Could you check a few things on this model? Use its own coordinates, in mm. A direction names the side the tool comes from. Round coordinates to 2 decimals unless told otherwise and drop trailing zeros. Loops run counter-clockwise (first coordinate to the right, second up) from the corner with the lowest first, then second, coordinate; pieces in that order, holes last. Notation, with made-up numbers: (29, -30.75) - (84, -30.75) arc R13 cw to (84, -26.75) - close; hole circle Ø2 at (83.5, -10.5). An arc over 180 degrees is marked (long way). Use one line per item in the form item = value.
```python
from build123d import *

# Parameters (mm, degrees)
F0_R     = 8.001
F0_R_2   = 1.27
F1_DEPTH = 31.75
F2_R     = 2.413
F2_R_2   = 1.27
F3_DEPTH = 19.05
F4_R     = 2.159
F5_DEPTH = 12.7
F6_DEPTH = 12.7


with BuildPart() as f1:
    # F0 (on Top) → F1 (new body)
    with BuildSketch(Plane.XY):
        Circle(F0_R)
        Circle(F0_R_2, mode=Mode.SUBTRACT)
    extrude(amount=F1_DEPTH)

    # F2 (on face) → F3 (cut)
    with BuildSketch(Plane.XY.offset(31.75)):
        Circle(F2_R)
        Circle(F2_R_2, mode=Mode.SUBTRACT)
    extrude(amount=-F3_DEPTH, mode=Mode.SUBTRACT)

    # F4 (on Right) → F5 (cut, symmetric)
    with BuildSketch(Plane.YZ):
        with Locations((0, 20.955)):
            Circle(F4_R)
    extrude(amount=F5_DEPTH, both=True, mode=Mode.SUBTRACT)

    # F4 (on Right) → F6 (cut, symmetric)
    with BuildSketch(Plane.YZ):
        with Locations((0, 6.35)):
            Circle(F4_R)
    extrude(amount=F6_DEPTH, both=True, mode=Mode.SUBTRACT)


solid = f1.part
```
1. Please list where these lines run through material, in increasing order: line 1 along Z through (x, y) = (6.75, 0); line 2 along Y through (x, z) = (0, 2.65).
Solution:
line_1 = 0 to 4.19, 8.51 to 18.8, 23.11 to 31.75
line_2 = -8 to -1.27, 1.27 to 8
2. We'd pull the mould along Y, two halves only. Please class faces 1 (the face through (1.04, -1.04, 12.7)), 2 (the face through (2, 0, 0)), 3 (the face through (-1.27, 0.06, 2.27)), 4 (the face through (7.632, 2.403, 15.653)): +Y half, -Y half, draft (parallel to the pull), parting line (faces both ways), or undercut.
Solution:
face_1 = undercut
face_2 = draft
face_3 = undercut
face_4 = parting line
3. If we section it at A-A, the plane y = 0: Write out the boundary of the cut face in (x, z), plus the area to 3 significant figures.
Solution:
outline = (-8, 0) - (-1.27, 0) - (-1.27, 4.19) - (-8, 4.19) - close; (-8, 8.51) - (-1.27, 8.51) - (-1.27, 12.7) - (-2.41, 12.7) - (-2.41, 18.8) - (-8, 18.8) - close; (-8, 23.11) - (-2.41, 23.11) - (-2.41, 31.75) - (-8, 31.75) - close; (1.27, 0) - (8, 0) - (8, 4.19) - (1.27, 4.19) - close; (1.27, 8.51) - (8, 8.51) - (8, 18.8) - (2.41, 18.8) - (2.41, 12.7) - (1.27, 12.7) - close; (2.41, 23.11) - (8, 23.11) - (8, 31.75) - (2.41, 31.75) - close
area = 277 mm^2
4. On a 3-axis mill with a long thin cutter (end or side, diameter ignored), from which of +Z, -Z, +X, -X, +Y, -Y can I reach the whole of each face in a straight line? I mean faces 5 (the face through (1.21, 0.38, 10.37)), 6 (the face through (1.113, -2.141, 22.358)). Say none if no direction works.
Solution:
face_5 = +Z, -Z
face_6 = +Z
5. For P1, Ø3, axis at x = -4.5, z = 17.5, coming from the +Y side; P2, Ø2, axis at y = 4, z = 24, coming from the +X side; P3, Ø1.4, axis at x = 0.5, y = -1, coming from the +Z side, each with a flat end and sliding along its axis, tell me the tip position at first contact or that it passes through.
Solution:
P1 = 7.42
P2 = 7.42
P3 = 12.7
6. If we section it at B-B, the plane x = 0: Write out the boundary of the cut face in (y, z).
Solution:
outline = (-8, 0) - (-1.27, 0) - (-1.27, 4.6) arc R2.16 cw to (-1.27, 8.1) - (-1.27, 12.7) - (-2.41, 12.7) - (-2.41, 31.75) - (-8, 31.75) - close; (1.27, 0) - (8, 0) - (8, 31.75) - (2.41, 31.75) - (2.41, 12.7) - (1.27, 12.7) - (1.27, 8.1) arc R2.16 cw to (1.27, 4.6) - close
7. If we section it at D-D, the plane z = 24: Write out the boundary of the cut face in (x, y), plus the area to 3 significant figures.
Solution:
outline = circle Ø16 at (0, 0); hole circle Ø4.83 at (0, 0)
area = 183 mm^2
8. If we section it at C-C, the plane x = 4.75: Write out the boundary of the cut face in (y, z) (3 decimals), plus the area to 3 significant figures.
Solution:
outline = (-6.438, 0) - (6.438, 0) - (6.438, 31.75) - (-6.438, 31.75) - close; hole circle Ø4.318 at (0, 6.35); hole circle Ø4.318 at (0, 20.955)
area = 380 mm^2
